The listing builds one solid part. Answer for the finished solid, in the listing's coordinates (mm). A direction names the side the tool comes from. Round coordinates to 2 decimals unless told otherwise and drop trailing zeros. Order: outer loops, then holes, each group sorted by start corner. A loop starts at its lowest first (then second) coordinate and runs counter-clockwise, first axis right, second up. Notation, with made-up numbers: (3.25, -3.5) - (40.25, -3.5) arc R8 cw to (40.25, 8.5) - close; hole circle Ø8 at (-4, 70). An arc over 180 degrees is marked (long way). One line per item, written item: value. Start each with the question number.
1. Flat-ended cylindrical pins translate along their axes: P1, Ø5.5, axis at y = -12, z = 125.5, coming from the +X side; P2, Ø9.5, axis at y = -10.5, z = 67, coming from the -X side; P3, Ø10, axis at x = -354, y = -4.5, coming from the -Z side (3 decimals). Find the tip coordinate at first contact, or state that the pin passes through.
2. Straight lines are drawn through the part: line 1 (Z direction, x = 256.5, y = -14) (3 decimals); line 2 (X direction, y = -9.75, z = 94); line 3 (Z direction, x = 142, y = -14.75) (3 decimals). For each, find the intervals that lie inside material, in ascending order.
3. Section B-B, the plane z = 95.5 is taken. Give the vertices of the cut face in (x, y).
4. Section A-A, the plane x = 227.5 is taken. Give the vertices of the cut face in (y, z) (3 decimals), then the cut area to 3 significant figures.
5. A tool of negligible diameter and unlimited length cuts with its end or side. For faces 1 (the flat face through (-448, -9, 66.675)), 2 (the flat face through (448, -9, 66.675)), 3 (the flat face through (438.15, -9, -153)), 4 (the flat face through (-438.15, -9, -151)), 5 (the flat face through (247, -9, 34.925)), from which of +Z, -Z, +X, -X, +Y, -Y can it reach the whole face along a straight path? Write none if from no direction.
6. Section D-D, the plane z = -201.5 is taken. Give the vertices of the cut face in (x, y).
7. Section C-C, the plane x = 380.5 is taken. Give the vertices of the cut face in (y, z) (3 decimals).
from build123d import *

# Parameters (mm, degrees)
F0_W     = 19.05
F0_H     = 152.4
F0_W_2   = 304.8
F0_H_2   = 38.1
F1_DEPTH = 19.05


# Not quite as in the source:
# - a feature names something its author has since deleted; it is built from what else it names


with BuildPart() as f1:
    # F0 (on Front) → F1 (new body)
    with BuildSketch(Plane.XZ):
        Polygon((438.15, 219.075), (-438.15, 219.075), (-438.15, 66.675), (-438.15, -85.725), (-438.15, -219.075), (-152.4, -219.075), (152.4, -219.075), (438.15, -219.075), (438.15, -85.725), (438.15, 66.675), align=None)
        Polygon((-304.8, 111.125), (304.8, 111.125), (304.8, 34.925), (304.8, -3.175), (285.75, -3.175), (285.75, 34.925), (206.375, 34.925), (206.375, -3.175), (187.325, -3.175), (187.325, 34.925), (107.95, 34.925), (107.95, -3.175), (88.9, -3.175), (88.9, 34.925), (9.525, 34.925), (9.525, -3.175), (-9.525, -3.175), (-9.525, 34.925), (-88.9, 34.925), (-88.9, -3.175), (-107.95, -3.175), (-107.95, 34.925), (-187.325, 34.925), (-187.325, -3.175), (-206.375, -3.175), (-206.375, 34.925), (-285.75, 34.925), (-285.75, -3.175), (-304.8, -3.175), (-304.8, 34.925), align=None, mode=Mode.SUBTRACT)
        with Locations((-447.675, -9.525)):
            Rectangle(F0_W, F0_H)
        with Locations((0, -238.125)):
            Rectangle(F0_W_2, F0_H_2)
        with Locations((447.675, -9.525)):
            Rectangle(F0_W, F0_H)
    extrude(amount=F1_DEPTH)


solid = f1.part
Answer list:
1. P1: stops at x = 438.15
1. P2: stops at x = -457.2
1. P3: stops at z = -219.075
2. line 1: z = -219.075 to 34.925, 111.125 to 219.075
2. line 2: x = -438.15 to -304.8, 304.8 to 438.15
2. line 3: z = -257.175 to 34.925, 111.125 to 219.075
3. outline: (-438.15, -19.05) - (-304.8, -19.05) - (-304.8, 0) - (-438.15, 0) - close; (304.8, -19.05) - (438.15, -19.05) - (438.15, 0) - (304.8, 0) - close
4. outline: (-19.05, -219.075) - (0, -219.075) - (0, 34.925) - (-19.05, 34.925) - close; (-19.05, 111.125) - (0, 111.125) - (0, 219.075) - (-19.05, 219.075) - close
4. area: 6,900 mm²
5. face 1: +Z, -X, +Y, -Y
5. face 2: +Z, +X, +Y, -Y
5. face 3: -Z, +X, +Y, -Y
5. face 4: -Z, -X, +Y, -Y
5. face 5: +Y, -Y
6. outline: (-438.15, -19.05) - (438.15, -19.05) - (438.15, 0) - (-438.15, 0) - close
7. outline: (-19.05, -219.075) - (0, -219.075) - (0, 219.075) - (-19.05, 219.075) - close
